Source: CAD feature listing. Evaluate the final solid. Frame: model axes, mm. A direction names the side the tool comes from. Round coordinates to 2 decimals unless told otherwise and drop trailing zeros. Loops run counter-clockwise (first coordinate to the right, second up) from the corner with the lowest first, then second, coordinate; pieces in that order, holes last. Notation, with made-up numbers: (0.25, -28) - (49.25, -28) arc R13 cw to (49.25, -22) - close; hole circle Ø2 at (9.5, 12.5). An arc over 180 degrees is marked (long way). One line per question, with ' | ' between items.
from build123d import *

# Parameters (mm, degrees)
SKETCH2_R           = 19
BOSS_EXTRUDE1_DEPTH = 1.3
BOSS_EXTRUDE7_START = -1.3
BOSS_EXTRUDE7_DEPTH = 1.3
SKETCH17_R          = 0.7
BOSS_EXTRUDE9_DEPTH = 1.3
BOSS_EXTRUDE2_START = -1.3
SKETCH3_R           = 35
SKETCH3_R_2         = 19
BOSS_EXTRUDE2_DEPTH = 1.3
SKETCH6_R           = 5
BOSS_EXTRUDE4_DEPTH = 1
SKETCH7_R           = 59.131365533
CUT_EXTRUDE1_DEPTH  = 10
FILLET1_R           = 6
SKETCH4_R           = 3.2
CUT_EXTRUDE2_DEPTH  = 10


with BuildPart() as part:
    # Sketch2 → Boss-Extrude1 (new body)
    with BuildSketch(Plane.XY.offset(10)):
        Circle(SKETCH2_R)
        with BuildLine():
            ThreePointArc((0, 0.943688479), (0.291615777, 0.897501077), (0.554686171, 0.763460017))
            Line((0.554686171, 0.763460017), (10.580134541, 14.562305899))
            ThreePointArc((10.580134541, 14.562305899), (14.562305899, 10.580134541), (17.119017293, 5.562305899))
            Line((17.119017293, 5.562305899), (0.897501077, 0.291615777))
            ThreePointArc((0.897501077, 0.291615777), (0.943688479, 0), (0.897501077, -0.291615777))
            Line((0.897501077, -0.291615777), (17.119017293, -5.562305899))
            ThreePointArc((17.119017293, -5.562305899), (14.562305899, -10.580134541), (10.580134541, -14.562305899))
            Line((10.580134541, -14.562305899), (0.554686171, -0.763460017))
            ThreePointArc((0.554686171, -0.763460017), (0.291615777, -0.897501077), (0, -0.943688479))
            Line((0, -0.943688479), (0, -18))
            ThreePointArc((0, -18), (-5.562305899, -17.119017293), (-10.580134541, -14.562305899))
            Line((-10.580134541, -14.562305899), (-0.554686171, -0.763460017))
            ThreePointArc((-0.554686171, -0.763460017), (-0.763460017, -0.554686171), (-0.897501077, -0.291615777))
            Line((-0.897501077, -0.291615777), (-17.119017293, -5.562305899))
            ThreePointArc((-17.119017293, -5.562305899), (-18, 0), (-17.119017293, 5.562305899))
            Line((-17.119017293, 5.562305899), (-0.897501077, 0.291615777))
            ThreePointArc((-0.897501077, 0.291615777), (-0.763460017, 0.554686171), (-0.554686171, 0.763460017))
            Line((-0.554686171, 0.763460017), (-10.580134541, 14.562305899))
            ThreePointArc((-10.580134541, 14.562305899), (-5.562305899, 17.119017293), (0, 18))
            Line((0, 18), (0, 0.943688479))
        make_face(mode=Mode.SUBTRACT)
        with BuildLine():
            Line((0.5, 1.198581445), (0.5, 17.492855685))
            ThreePointArc((0.5, 17.492855685), (5.50283957, 16.612307385), (10.042025258, 14.332052495))
            Line((10.042025258, 14.332052495), (0.5, 1.198581445))
        make_face(mode=Mode.SUBTRACT)
        with BuildLine():
            Line((-0.985410197, 0.845910294), (-16.48218589, 5.881117945))
            ThreePointArc((-16.48218589, 5.881117945), (-14.098772245, 10.366996729), (-10.527435455, 13.979381344))
            Line((-10.527435455, 13.979381344), (-0.985410197, 0.845910294))
        make_face(mode=Mode.SUBTRACT)
        with BuildLine():
            Line((-1.109016994, -0.675780132), (-10.686551089, -13.858124903))
            ThreePointArc((-10.686551089, -13.858124903), (-14.216360017, -10.205151045), (-16.548338183, -5.692319683))
            Line((-16.548338183, -5.692319683), (-1.109016994, -0.675780132))
        make_face(mode=Mode.SUBTRACT)
        with BuildLine():
            ThreePointArc((9.877534095, -14.445910155), (5.312578558, -16.674126936), (0.3, -17.497428382))
            Line((0.3, -17.497428382), (0.3, -1.263565384))
            Line((0.3, -1.263565384), (9.877534095, -14.445910155))
        make_face(mode=Mode.SUBTRACT)
        with BuildLine():
            Line((16.73374838, -5.121685773), (1.294427191, -0.105146222))
            Line((1.294427191, -0.105146222), (16.791202885, 4.930061429))
            ThreePointArc((16.791202885, 4.930061429), (17.499714134, -0.100026134), (16.73374838, -5.121685773))
        make_face(mode=Mode.SUBTRACT)
    extrude(amount=-BOSS_EXTRUDE1_DEPTH)

    # Sketch11 → Boss-Extrude7 (add)
    with BuildSketch(Plane(origin=(0, 0, 8.7), x_dir=(-1, 0, 0), z_dir=(0, 0, -1)).offset(BOSS_EXTRUDE7_START)):
        with BuildLine():
            ThreePointArc((-0.897501077, 0.291615777), (-0.763460017, 0.554686171), (-0.554686171, 0.763460017))
            Line((-0.554686171, 0.763460017), (-10.580134541, 14.562305899))
            ThreePointArc((-10.580134541, 14.562305899), (-14.562305899, 10.580134541), (-17.119017293, 5.562305899))
            Line((-17.119017293, 5.562305899), (-0.897501077, 0.291615777))
        make_face()
        with BuildLine():
            Line((0, 18), (0, 0.943688479))
            ThreePointArc((0, 0.943688479), (0.291615777, 0.897501077), (0.554686171, 0.763460017))
            Line((0.554686171, 0.763460017), (10.580134541, 14.562305899))
            ThreePointArc((10.580134541, 14.562305899), (5.562305899, 17.119017293), (0, 18))
        make_face()
        with BuildLine():
            Line((17.119017293, 5.562305899), (0.897501077, 0.291615777))
            ThreePointArc((0.897501077, 0.291615777), (0.932070108, 0.147625402), (0.943688479, 0))
            ThreePointArc((0.943688479, 0), (0.932070108, -0.147625402), (0.897501077, -0.291615777))
            Line((0.897501077, -0.291615777), (17.119017293, -5.562305899))
            ThreePointArc((17.119017293, -5.562305899), (18, 0), (17.119017293, 5.562305899))
        make_face()
        with BuildLine():
            Line((10.580134541, -14.562305899), (0.554686171, -0.763460017))
            ThreePointArc((0.554686171, -0.763460017), (0.291615777, -0.897501077), (0, -0.943688479))
            Line((0, -0.943688479), (0, -18))
            ThreePointArc((0, -18), (5.562305899, -17.119017293), (10.580134541, -14.562305899))
        make_face()
        with BuildLine():
            ThreePointArc((-0.554686171, -0.763460017), (-0.763460017, -0.554686171), (-0.897501077, -0.291615777))
            Line((-0.897501077, -0.291615777), (-17.119017293, -5.562305899))
            ThreePointArc((-17.119017293, -5.562305899), (-14.562305899, -10.580134541), (-10.580134541, -14.562305899))
            Line((-10.580134541, -14.562305899), (-0.554686171, -0.763460017))
        make_face()
        with BuildLine():
            ThreePointArc((0.554686171, 0.763460017), (0.291615777, 0.897501077), (0, 0.943688479))
            ThreePointArc((0, 0.943688479), (-0.291615777, 0.897501077), (-0.554686171, 0.763460017))
            ThreePointArc((-0.554686171, 0.763460017), (-0.763460017, 0.554686171), (-0.897501077, 0.291615777))
            ThreePointArc((-0.897501077, 0.291615777), (-0.943688479, 0), (-0.897501077, -0.291615777))
            ThreePointArc((-0.897501077, -0.291615777), (-0.763460017, -0.554686171), (-0.554686171, -0.763460017))
            ThreePointArc((-0.554686171, -0.763460017), (-0.291615777, -0.897501077), (0, -0.943688479))
            ThreePointArc((0, -0.943688479), (0.291615777, -0.897501077), (0.554686171, -0.763460017))
            ThreePointArc((0.554686171, -0.763460017), (0.763460017, -0.554686171), (0.897501077, -0.291615777))
            ThreePointArc((0.897501077, -0.291615777), (0.932070108, -0.147625402), (0.943688479, 0))
            ThreePointArc((0.943688479, 0), (0.932070108, 0.147625402), (0.897501077, 0.291615777))
            ThreePointArc((0.897501077, 0.291615777), (0.763460017, 0.554686171), (0.554686171, 0.763460017))
        make_face()
    extrude(amount=BOSS_EXTRUDE7_DEPTH)

    # Sketch17 → Boss-Extrude9 (add)
    with BuildSketch(Plane(origin=(0, 0, 8.7), x_dir=(-1, 0, 0), z_dir=(0, 0, -1))):
        Circle(SKETCH17_R)
    extrude(amount=-BOSS_EXTRUDE9_DEPTH)

    # Sketch3 → Boss-Extrude2 (add)
    with BuildSketch(Plane(origin=(0, 0, 8.7), x_dir=(-1, 0, 0), z_dir=(0, 0, -1)).offset(BOSS_EXTRUDE2_START)):
        Circle(SKETCH3_R)
        Circle(SKETCH3_R_2, mode=Mode.SUBTRACT)
    extrude(amount=BOSS_EXTRUDE2_DEPTH)

    # Sketch6 → Boss-Extrude4 (add)
    with BuildSketch(Plane(origin=(0, 0, 10), x_dir=(-1, 0, 0), z_dir=(0, 0, -1))):
        with Locations((0, 30)):
            Circle(SKETCH6_R)
        with Locations((25.980762114, -15)):
            Circle(SKETCH6_R)
        with Locations((-25.980762114, -15)):
            Circle(SKETCH6_R)
    extrude(amount=BOSS_EXTRUDE4_DEPTH)

    # Sketch7 → Cut-Extrude1 (cut)
    with BuildSketch(Plane(origin=(0, 0, 8.7), x_dir=(-1, 0, 0), z_dir=(0, 0, -1))):
        Circle(SKETCH7_R)
        Polygon((0, 42), (-36.373066959, -21), (36.373066959, -21), align=None, mode=Mode.SUBTRACT)
    extrude(amount=-CUT_EXTRUDE1_DEPTH, mode=Mode.SUBTRACT)

    # Fillet1
    fillet1_edges = [part.edges().sort_by_distance(p)[0] for p in [
        (4.186533479, 34.748711306, 9.35),
        (32.186533479, -13.748711306, 9.35),
        (28, -21, 9.35),
        (-28, -21, 9.35),
        (-32.186533479, -13.748711306, 9.35),
        (-4.186533479, 34.748711306, 9.35),
    ]]
    fillet(fillet1_edges, radius=FILLET1_R)

    # Sketch4 → Cut-Extrude2 (cut)
    with BuildSketch(Plane(origin=(0, 0, 8.7), x_dir=(-1, 0, 0), z_dir=(0, 0, -1))):
        with Locations((0, 29)):
            Circle(SKETCH4_R)
        with Locations((25.11473671, -14.5)):
            Circle(SKETCH4_R)
        with Locations((-25.11473671, -14.5)):
            Circle(SKETCH4_R)
    extrude(amount=-CUT_EXTRUDE2_DEPTH, mode=Mode.SUBTRACT)


solid = part.part
1. Section query C-C, the plane x = 23.5. Return loops of the section in (y, z).
Worked out:
outline: (-21, 8.7) - (-17.26, 8.7) - (-17.26, 10) - (-21, 10) - close; (-11.74, 8.7) - (1.3, 8.7) - (1.3, 10) - (-11.74, 10) - close
2. Section query A-A, the plane z = 9.55. Give the number of separate pieces and of enclosed holes in the cut face, plus the area to 3 significant figures.
Worked out:
separate pieces: 1 | enclosed holes: 8 | area: 1,680 mm2
3. Section query B-B, the plane y = 29. Return loops of the section in (x, z), plus the area to 3 significant figures.
Worked out:
outline: (-7.51, 8.7) - (-3.2, 8.7) - (-3.2, 10) - (-7.51, 10) - close; (3.2, 8.7) - (7.51, 8.7) - (7.51, 10) - (3.2, 10) - close | area: 11.2 mm2
4. Access query for faces 1 (the cylindrical face through (-27.805, -20.205, 9.359)), 2 (the flat face through (-5.831, -7.175, 9.359)). Directions: +Z, -Z, +X, -X, +Y, -Y. A direction counts if a zero-diameter tool reaches every point of the face in a straight line with its end or side. Return the directions, or none.
Worked out:
face 1: +Z, -Z, -X, -Y | face 2: +Z, -Z
5. Section query D-D, the plane y = 13. Return loops of the section in (x, z).
Worked out:
outline: (-16.74, 8.7) - (-11.72, 8.7) - (-11.72, 10) - (-16.74, 10) - close; (-9.82, 8.7) - (0.5, 8.7) - (0.5, 10) - (-9.82, 10) - close; (9.07, 8.7) - (16.74, 8.7) - (16.74, 10) - (9.07, 10) - close
6. Mould query, pull axis Y, two halves, no side actions, for faces 3 (the cylindrical face through (27.65, -16.45, 9.34)), 4 (the cylindrical face through (-3.6, 34.18, 9.36)), 5 (the cylindrical face through (-31.4, -14, 9.4)), 6 (the cylindrical face through (5.435, 16.635, 9.359)). Classes: released by +Y, released by -Y, zero draft, split by the parting line, or undercut.
Worked out:
face 3: undercut | face 4: released by +Y | face 5: split by the parting line | face 6: undercut
7. Material intervals for probe 1 along Y at (x, z) = (0, 9.6); probe 2 along Y at (x, z) = (-4.5, 9.45); probe 3 along X at (y, z) = (-12, 9), sorted ascending.
Worked out:
probe 1: y = -21 to 25.8, 32.2 to 35 | probe 2: y = -21 to -5.34, -1.78 to 1.99, 5.68 to 33.54 | probe 3: x = -31.06 to -27.11, -23.12 to -12.74, -9.34 to 0.3, 8.1 to 23.12, 27.11 to 31.06
